Read the model definition and answer for the solid it produces. Units are mm, in the model's axes. Face numbers are marked on the shaded views. Round coordinates to 2 decimals unless told otherwise and drop trailing zeros. Order: outer loops, then holes, each group sorted by start corner. A loop starts at its lowest first (then second) coordinate and runs counter-clockwise, first axis right, second up. Notation, with made-up numbers: (34, 10.5) -> (63, 10.5) arc R14 cw to (63, 31.5) -> close; hole circle Ø2 at (15, 32). An arc over 180 degrees is marked (long way). Answer as a JSON object with one key per item and string values. Group by question number.
Item 1: Section D-D, the plane z = 13 is taken. Write down the section's boundary in (x, y) (3 decimals), plus the area to 3 significant figures.
Item 2: Section C-C, the plane z = 21 is taken. Write down the section's boundary in (x, y) (3 decimals), plus the area to 3 significant figures.
Item 3: Section A-A, the plane y = -78 is taken. Write down the section's boundary in (x, z) (3 decimals), plus the area to 3 significant figures.
Item 4: Section B-B, the plane x = -3.5 is taken. Write down the section's boundary in (y, z), plus the area to 3 significant figures.
Item 5: Given P1, Ø1.5, axis at y = -37.5, z = 36, coming from the -X side; P2, Ø4, axis at y = -68, z = 44, coming from the -X side; P3, Ø1.5, axis at y = -25.5, z = 34, coming from the -X side; P4, Ø19, axis at x = 0, z = 31.75, coming from the +Y side, each flat-ended and moving along its own axis, determine where each tip first touches the part or whether it passes through.
Item 6: Consider probe 1 along Z at (x, y) = (0, -28) (3 decimals); probe 2 along X at (y, z) = (-18, 31) (3 decimals); probe 3 along X at (y, z) = (-63, 25) (3 decimals). Determine where each line is inside the solid, lowest interval first. Write a range as from..to.
Item 7: The mould has two halves that part along Z. Classify the marked faces 1, 2 and 3: pulls with the +Z half, pulls with the -Z half, needs draft (parallel to the pull), parting line crosses it, or undercut.
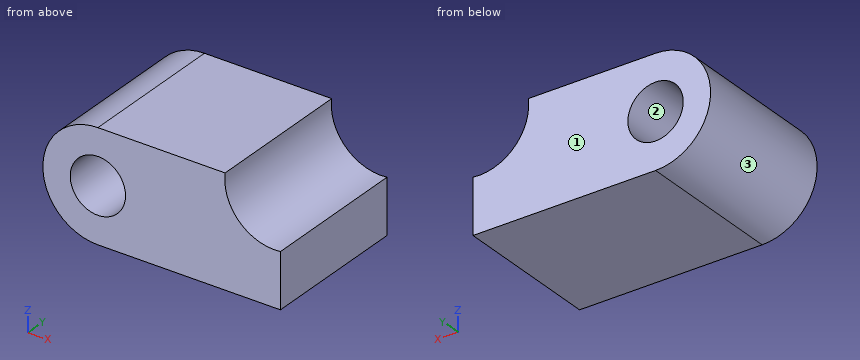
from build123d import *

# Parameters (mm, degrees)
F0_R     = 15.875
F1_DEPTH = 85.598


with BuildPart() as f1:
    # F0 (on Front) → F1 (new body)
    with BuildSketch(Plane.XZ):
        with BuildLine():
            ThreePointArc((0, 63.131541), (-31.565771, 31.565771), (0, 0))
            Line((0, 0), (104.775, 0))
            Line((104.775, 0), (104.775, 31.381541))
            ThreePointArc((104.775, 31.381541), (81.194411, 39.550952), (73.025, 63.131541))
            Line((73.025, 63.131541), (0, 63.131541))
        make_face()
        with Locations((0, 31.75)):
            Circle(F0_R, mode=Mode.SUBTRACT)
    extrude(amount=F1_DEPTH)


solid = f1.part
Values found:
{
 "1": {"outline": "(-25.529, -85.598) -> (104.775, -85.598) -> (104.775, 0) -> (-25.529, 0) -> close", "area": "11,200 mm2"},
 "2": {"outline": "(-29.745, -85.598) -> (-11.681, -85.598) -> (-11.681, 0) -> (-29.745, 0) -> close; (11.681, -85.598) -> (104.775, -85.598) -> (104.775, 0) -> (11.681, 0) -> close", "area": "9,510 mm2"},
 "3": {"outline": "(0, 0) -> (104.775, 0) -> (104.775, 31.382) arc R28.575 cw to (73.025, 63.132) -> (0, 63.132) arc R31.566 ccw to start; hole circle Ø31.75 at (0, 31.75)", "area": "6,540 mm2"},
 "4": {"outline": "(-85.6, 0.19) -> (0, 0.19) -> (0, 16.27) -> (-85.6, 16.27) -> close; (-85.6, 47.23) -> (0, 47.23) -> (0, 62.94) -> (-85.6, 62.94) -> close", "area": "2,720 mm2"},
 "5": {"P1": "x = -31.35", "P2": "x = -29.79", "P3": "x = -31.52", "P4": "through"},
 "6": {"probe 1": "0..15.875, 47.625..63.132", "probe 2": "-31.561..-15.857, 15.857..104.775", "probe 3": "-30.875..-14.368, 14.368..104.775"},
 "7": {"face 1": "needs draft", "face 2": "undercut", "face 3": "parting line crosses it"}
}
